Here's the drawing with two shaded views (mm, measured from the low corner). I have some questions. Round coordinates to 2 decimals unless told otherwise and drop trailing zeros. Order: outer loops, then holes, each group sorted by start corner. A loop starts at its lowest first (then second) coordinate and runs counter-clockwise, first axis right, second up.
Q1. If we section it at A-A (y = 34): Please give me the cut outline in (x, z).
Q2. Will these pins go through, and if not, where does the flat tip stop? P1, Ø0.6, axis at y = 3.5, z = 26, coming from the +X side; P2, Ø1.6, axis at y = 56, z = 26, coming from the -X side; P3, Ø0.6, axis at x = 55.5, z = 17, coming from the +Y side; P4, Ø9, axis at x = 30, y = 30, coming from the +Z side.
Q3. We'd pull the mould along X, two halves only. Please class the marked faces 1, 2 and 3: pulls with the +X half, pulls with the -X half, needs draft (parallel to the pull), parting line crosses it, or undercut.
Q4. If I drill on line 1 (Y direction, x = 30, z = 29); line 2 (Y direction, x = 3, z = 22); line 3 (X direction, y = 31, z = 53.5), over which ranges is the centre line in solid material (lowest first)?
Q5. If we section it at C-C (z = 39.5): Please give me the cut outline in (x, y), plus the area to 3 significant figures.
Q6. If we section it at B-B (x = 30): Please give me the cut outline in (y, z).
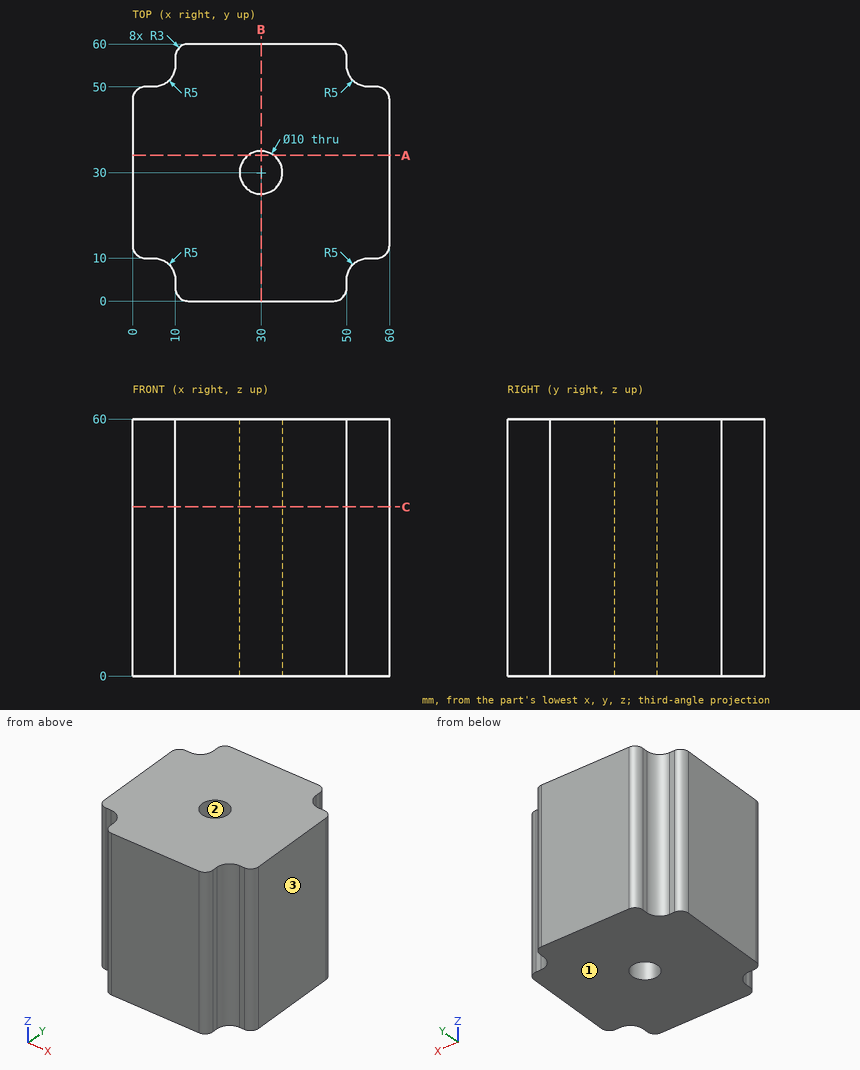
Solution:
1. outline: (0, 0) - (27, 0) - (27, 60) - (0, 60) - close; (33, 0) - (60, 0) - (60, 60) - (33, 60) - close
2. P1: stops at x = 50
2. P2: stops at x = 10
2. P3: stops at y = 50
2. P4: passes through
3. face 1: needs draft
3. face 2: undercut
3. face 3: pulls with the +X half
4. line 1: y = 0 to 25, 35 to 60
4. line 2: y = 10 to 50
4. line 3: x = 0 to 25.1, 34.9 to 60
5. outline: (0, 13) arc R3 ccw to (3, 10) - (5, 10) arc R5 cw to (10, 5) - (10, 3) arc R3 ccw to (13, 0) - (47, 0) arc R3 ccw to (50, 3) - (50, 5) arc R5 cw to (55, 10) - (57, 10) arc R3 ccw to (60, 13) - (60, 47) arc R3 ccw to (57, 50) - (55, 50) arc R5 cw to (50, 55) - (50, 57) arc R3 ccw to (47, 60) - (13, 60) arc R3 ccw to (10, 57) - (10, 55) arc R5 cw to (5, 50) - (3, 50) arc R3 ccw to (0, 47) - close; hole circle Ø10 at (30, 30)
5. area: 3,130 mm2
6. outline: (0, 0) - (25, 0) - (25, 60) - (0, 60) - close; (35, 0) - (60, 0) - (60, 60) - (35, 60) - close
